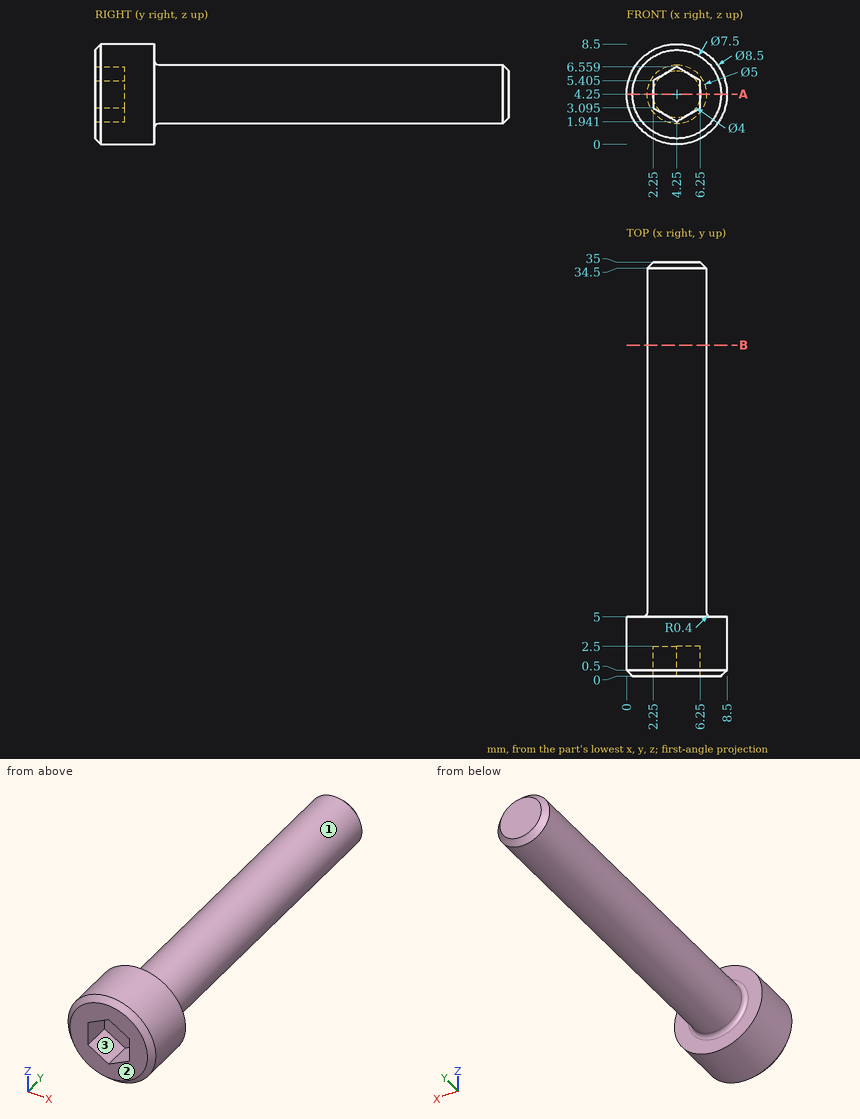
Can you work these out from the drawing? Everything is in mm from the part's minimum corner. Coordinates: 2 decimals unless noted, no trailing zeros. Write each loop counter-clockwise with the first axis right and the second up, starting at its lowest first coordinate (ties: lowest second). Pieces come first, ordered by that corner, then holes. Notation, with made-up numbers: (-20.5, -37.5) -> (-14.5, -37.5) arc R17 cw to (-14.5, -19.5) -> close; hole circle Ø11 at (-25, -35.75). An arc over 180 degrees is marked (long way). Write item = value, one per line.
(1) Imagine slicing it at B-B (y = 28). Please give me the cut outline in (x, z), and give its area (3 significant figures).
Verdict:
outline = circle Ø5 at (4.25, 4.25)
area = 19.6 mm^2
(2) Thinking about a two-plate mould opening in X: for the marked faces 1, 2 and 3, which applies, +X half, -X half, draft (parallel to the pull), parting line (faces both ways), or undercut?
Verdict:
face_1 = parting line
face_2 = draft
face_3 = undercut
(3) For pin 1 (1 mm diameter, centred on y = 8.5, z = 2.5, fed in from +X) (1 decimal); pin 2 (1.2 mm diameter, centred on x = 4.5, z = 3, fed in from -Y); pin 3 (4 mm diameter, centred on x = 7.5, y = 14.5, fed in from -Z) (1 decimal), each with a flat end and sliding along its axis, tell me the tip position at first contact or that it passes through.
Verdict:
pin_1 = 6.4
pin_2 = 2.5
pin_3 = 2.1
(4) Imagine slicing it at A-A (z = 4.25). Please give me the cut outline in (x, y), and give its area (3 significant figures).
Verdict:
outline = (0, 0.5) -> (0.5, 0) -> (2.25, 0) -> (2.25, 2.5) -> (6.25, 2.5) -> (6.25, 0) -> (8, 0) -> (8.5, 0.5) -> (8.5, 5) -> (7.15, 5) arc R0.4 cw to (6.75, 5.4) -> (6.75, 34.5) -> (6.25, 35) -> (2.25, 35) -> (1.75, 34.5) -> (1.75, 5.4) arc R0.4 cw to (1.35, 5) -> (0, 5) -> close
area = 182 mm^2
(5) If I drill on probe 1 along Y at (x, z) = (2.25, 1.25); probe 2 along Y at (x, z) = (2.5, 3.5); probe 3 along Z at (x, y) = (0.5, 2.5), over which ranges is the centre line in solid material (lowest first)?
Verdict:
probe_1 = 0 to 5
probe_2 = 2.5 to 35
probe_3 = 2.25 to 6.25
